```python
from build123d import *

# Parameters (mm, degrees)
CYLINDER006_R            = 1.6
CYLINDER006_DEPTH        = 10
BOX005_W                 = 5
BOX005_H                 = 145
BOX005_DEPTH             = 5
CLONE001_PLACEMENT_ANGLE = 90
BOX003_W                 = 8
BOX003_H                 = 8
BOX003_DEPTH             = 20
ARRAY001_X_COUNT         = 3
ARRAY001_X_PITCH         = 50
ARRAY001_Y_COUNT         = 3
ARRAY001_Y_PITCH         = 50
BOX002_W                 = 150
BOX002_H                 = 190
BOX002_DEPTH             = 3
CLONE002_PLACEMENT_ANGLE = 90
CHAMFER_SIZE             = 2


with BuildPart() as cylinder006:
    # Cylinder006 → Cylinder006 (new body)
    with BuildSketch(Plane(origin=(-9, 169, 6.3), x_dir=(1, 0, 0), z_dir=(0, 0, 1))):
        Circle(CYLINDER006_R)
    extrude(amount=CYLINDER006_DEPTH)


with BuildPart() as clone_of_cylinder007:
    # Clone007 base: copy of Cylinder006
    add(cylinder006.part)


with BuildPart() as clone_of_cylinder007_1:
    # Clone007 placement: moved
    add(clone_of_cylinder007.part.moved(Location((138, 0, 0))))


with BuildPart() as clone_of_cylinder006:
    # Clone006 base: copy of Cylinder006
    add(cylinder006.part)


with BuildPart() as clone_of_cylinder006_1:
    # Clone006 placement: moved
    add(clone_of_cylinder006.part.moved(Location((138, -178, 0))))


with BuildPart() as clone_of_fusion007:
    # Clone008 base: copy of Cylinder006
    add(cylinder006.part)


with BuildPart() as clone_of_fusion007_1:
    # Clone008 placement: moved
    add(clone_of_fusion007.part.moved(Location((0, -178, 0))))

    # Fusion007: union Clone of Cylinder007, Clone of Cylinder006, Cylinder006
    add(clone_of_cylinder007_1.part)
    add(clone_of_cylinder006_1.part)
    add(cylinder006.part)


with BuildPart() as clone_of_fusion007_2:
    # Clone009 placement: moved
    add(clone_of_fusion007_1.part.moved(Location((0, 0, 5))))


with BuildPart() as cube005:
    # Box005 → Box005 (new body)
    with BuildSketch(Plane(origin=(82.5, -12.5, 19.3), x_dir=(1, 0, 0), z_dir=(0, 0, 1))):
        with Locations((2.5, 72.5)):
            Rectangle(BOX005_W, BOX005_H)
    extrude(amount=BOX005_DEPTH)


with BuildPart() as clone_of_cube006:
    # Clone001 base: copy of Cube005
    add(cube005.part)


with BuildPart() as clone_of_cube006_1:
    # Clone001 placement: moved
    add(clone_of_cube006.part.moved(Location((120, 0, 0))).rotate(Axis((120, 0, 0), (0, 0, 1)), CLONE001_PLACEMENT_ANGLE))


with BuildPart() as clone_of_cube005:
    # Clone base: copy of Cube005
    add(cube005.part)


with BuildPart() as clone_of_cube005_1:
    # Clone placement: moved
    add(clone_of_cube005.part.moved(Location((-50, 0, 0))))


with BuildPart() as array001:
    # Box003 → Box003 (new body)
    with BuildSketch(Plane(origin=(6, 6, 5), x_dir=(1, 0, 0), z_dir=(0, 0, 1))):
        with Locations((4, 4)):
            Rectangle(BOX003_W, BOX003_H)
    extrude(amount=BOX003_DEPTH)

    # Array001 X: Array001 ×3


with BuildPart() as array001_1:
    add(array001.part)
    with Locations(*[(i * ARRAY001_X_PITCH, 0, 0) for i in range(1, ARRAY001_X_COUNT)]):
        add(array001.part)

    # Array001 Y: Array001 ×3


with BuildPart() as array001_2:
    add(array001_1.part)
    with Locations(*[(0, i * ARRAY001_Y_PITCH, 0) for i in range(1, ARRAY001_Y_COUNT)]):
        add(array001_1.part)


with BuildPart() as cut:
    # Box002 → Box002 (new body)
    with BuildSketch(Plane(origin=(-15, -15, 16.3), x_dir=(1, 0, 0), z_dir=(0, 0, 1))):
        with Locations((75, 95)):
            Rectangle(BOX002_W, BOX002_H)
    extrude(amount=BOX002_DEPTH)

    # Cut: cut Array001
    add(array001_2.part, mode=Mode.SUBTRACT)


with BuildPart() as chamfer_body:
    # Clone002 base: copy of Cube005
    add(cube005.part)


with BuildPart() as chamfer_body_1:
    # Clone002 placement: moved
    add(chamfer_body.part.moved(Location((120, -50, 0))).rotate(Axis((120, -50, 0), (0, 0, 1)), CLONE002_PLACEMENT_ANGLE))

    # Fusion005: union Clone of Cube006, Clone of Cube005, Cube005, Cut
    add(clone_of_cube006_1.part)
    add(clone_of_cube005_1.part)
    add(cube005.part)
    add(cut.part)

    # Cut005: cut Clone of Fusion007
    add(clone_of_fusion007_2.part, mode=Mode.SUBTRACT)

    # Chamfer
    chamfer_edges = [chamfer_body_1.edges().sort_by_distance(p)[0] for p in [
        (127.4, -9, 19.3),
        (-10.6, -9, 19.3),
        (127.4, 169, 19.3),
        (-10.6, 169, 19.3),
    ]]
    chamfer(chamfer_edges, length=CHAMFER_SIZE)


solid = chamfer_body_1.part
```
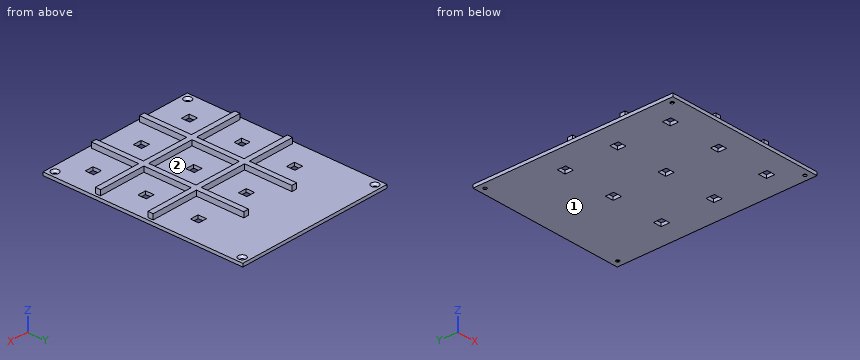
Work out the finished part from the listing and answer in its coordinate system (mm). Face numbers are marked on the shaded views. Give positions to 0.01 mm unless a question says otherwise; leave off trailing zeros. Order: outer loops, then holes, each group sorted by start corner. A loop starts at its lowest first (then second) coordinate and runs counter-clockwise, first axis right, second up.
1. Straight lines are drawn through the part: L1, parallel to X at y = -9, z = 17.05; L2, parallel to Y at x = 129, z = 16.75; L3, parallel to Y at x = 116, z = 23.5. For each, find the intervals that lie inside material, in ascending order.
Result sheet:
L1: x = -15 to -10.6, -7.4 to 127.4, 130.6 to 135
L2: y = -15 to -10.6, -7.4 to 167.4, 170.6 to 175
L3: y = 32.5 to 37.5, 82.5 to 87.5
2. Section A-A, the plane y = 61 is taken. Determine the outline of the cut face in (x, z), and give its area (3 significant figures).
Result sheet:
outline: (-15, 16.3) - (6, 16.3) - (6, 19.3) - (-15, 19.3) - close; (14, 16.3) - (56, 16.3) - (56, 19.3) - (37.5, 19.3) - (37.5, 24.3) - (32.5, 24.3) - (32.5, 19.3) - (14, 19.3) - close; (64, 16.3) - (106, 16.3) - (106, 19.3) - (87.5, 19.3) - (87.5, 24.3) - (82.5, 24.3) - (82.5, 19.3) - (64, 19.3) - close; (114, 16.3) - (135, 16.3) - (135, 19.3) - (114, 19.3) - close
area: 428 mm2
3. Each of these flat-tipped pins is pushed along its axis until it touches: P1, Ø1.5, axis at y = 104, z = 20.5, coming from the -X side; P2, Ø5, axis at x = -9, y = -9, coming from the +Z side; P3, Ø2.5, axis at y = 85, z = 22.5, coming from the -X side. Where does it stop, or does it pass through?
Result sheet:
P1: stops at x = 32.5
P2: stops at z = 18.2
P3: stops at x = -12.5
4. Section D-D, the plane x = 24.5 is taken. Determine the outline of the cut face in (y, z).
Result sheet:
outline: (-15, 16.3) - (175, 16.3) - (175, 19.3) - (87.5, 19.3) - (87.5, 24.3) - (82.5, 24.3) - (82.5, 19.3) - (37.5, 19.3) - (37.5, 24.3) - (32.5, 24.3) - (32.5, 19.3) - (-15, 19.3) - close
5. The mould has two halves that part along X. Classify the marked faces 1 and 2: released by +X, released by -X, zero draft, split by the parting line, or undercut.
Result sheet:
face 1: zero draft
face 2: undercut
6. Section C-C, the plane x = 9 is taken. Determine the outline of the cut face in (y, z), and give its area (3 significant figures).
Result sheet:
outline: (-15, 16.3) - (6, 16.3) - (6, 19.3) - (-15, 19.3) - close; (14, 16.3) - (56, 16.3) - (56, 19.3) - (37.5, 19.3) - (37.5, 24.3) - (32.5, 24.3) - (32.5, 19.3) - (14, 19.3) - close; (64, 16.3) - (106, 16.3) - (106, 19.3) - (87.5, 19.3) - (87.5, 24.3) - (82.5, 24.3) - (82.5, 19.3) - (64, 19.3) - close; (114, 16.3) - (175, 16.3) - (175, 19.3) - (114, 19.3) - close
area: 548 mm2
